Design review of the part built by this model. Coordinates are the model's own, in mm. Round coordinates to 2 decimals unless told otherwise and drop trailing zeros. One line per question, with ' | ' between items. Start each with the question number.
Item 1: Draft analysis for pull direction Z (two halves, no side actions). For faces 1 (the face through (-3, 7, 0)), 2 (the face through (-3, 7, -4.496)), state which applies: released by +Z, released by -Z, zero draft, split by the parting line, or undercut.
Item 2: Add section A-A, the plane z = -2.5. Give the number of separate pieces and of enclosed holes in the cut face, and give its area (3 significant figures).
Item 3: For L1, parallel to X at y = 142.5, z = -1.7; L2, parallel to Y at x = -160, z = -1.8; L3, parallel to X at y = 141.5, z = -2.8, list the stretches that pass through material, from the lowest coordinate up.
Autodesk Inventor part; units mm, degrees
ref_plane "YZ Plane" through (0, 0, 0) normal (1, 0, 0) x (0, 1, 0)
ref_plane "XZ Plane" through (0, 0, 0) normal (0, 1, 0) x (-1, 0, 0)
ref_plane "XY Plane" through (0, 0, 0) normal (0, 0, 1) x (1, 0, 0)
sketch "Sketch1" plane through (0, 0, 0) normal (0, 0, 1) x (1, 0, 0)
  line L0 (0, 316.484) -> (0, -316.484)
  line L1 (-334.6907, 0) -> (334.6907, 0)
  line L2 (239.0648, -226.06) -> (-239.0648, -226.06)
  line L3 (-239.0648, -226.06) -> (-239.0648, 226.06)
  line L4 (-239.0648, 226.06) -> (239.0648, 226.06)
  line L5 (239.0648, 226.06) -> (239.0648, -226.06)
  line L6 (239.0648, -226.06) -> (-239.0648, 226.06) construction
  line L7 (-239.0648, -226.06) -> (239.0648, 226.06) construction
  line L8 (220.345, -207.3402) -> (-220.345, -207.3402) construction
  line L9 (-220.345, -207.3402) -> (-220.345, 207.3402) construction
  line L10 (-220.345, 207.3402) -> (220.345, 207.3402) construction
  line L11 (220.345, 207.3402) -> (220.345, -207.3402) construction
  line L12 (220.345, -207.3402) -> (-220.345, 207.3402) construction
  line L13 (-220.345, -207.3402) -> (220.345, 207.3402) construction
  line L14 (-239.0648, -218.44) -> (239.0648, -218.44)
  line L15 (50.8, -191.06) -> (-50.8, -191.06)
  line L16 (-50.8, -191.06) -> (-50.8, -218.44)
  line L17 (-50.8, -218.44) -> (50.8, -218.44)
  line L18 (50.8, -218.44) -> (50.8, -191.06)
  line L19 (50.8, -191.06) -> (-50.8, -218.44) construction
  line L20 (-50.8, -191.06) -> (50.8, -218.44) construction
  point P0 (0, 0)
  point P1 (-156.5148, 207.3402)
  point P2 (0, 207.3402)
  point P3 (156.5148, 207.3402)
  point P4 (-156.5148, -207.3402)
  point P5 (0, -207.3402)
  point P6 (156.5148, -207.3402)
  point P7 (-220.345, 143.51)
  point P8 (-220.345, -143.51)
  point P9 (220.345, 143.51)
  point P10 (220.345, -117.0967)
  point P11 (-220.345, 0)
  point P12 (0, -218.44)
  point P13 (0, -226.06)
  point P14 (0, -204.75)
  point P15 (50.8, -218.44)
  dimension "d0" = 478.1296
  dimension "d1" = 452.12
  dimension "d3" = 18.7198
  dimension "d4" = 18.7198
  dimension "d7" = 143.51
  dimension "d8" = 143.51
  dimension "d10" = 82.55
  dimension "d20" = 82.55
  dimension "d21" = 82.55
  dimension "d23" = 7.62
  dimension "d24" = 35
  dimension "d25" = 101.6
extrude "Extrusion1" add sketch "Sketch1" against normal blind 4.4958 contours L4 L5 L1 L0 | L0 L1 L3 L4 | L1 L5 L14 L18 L15 L0 | L0 L15 L16 L14 L3 L1
hole "Hole1" at (-156.5148, 207.3402, 0) at (156.5148, 207.3402, 0) at (-156.5148, -207.3402, 0) at (156.5148, -207.3402, 0) at (220.345, 143.51, 0) at (220.345, -117.0967, 0) at (-220.345, 143.51, 0) at (-220.345, -143.51, 0) direction (0, 0, -1) diameter 8.255 end through all
fillet "Fillet1" radius 9.525 2 edges at (-239.0648, 226.06, -2.2479) (239.0648, 226.06, -2.2479)
fillet "Fillet2" radius 9.525 2 edges at (-239.0648, -218.44, -2.2479) (239.0648, -218.44, -2.2479)
fillet "Fillet3" radius 3.175 4 edges at (50.8, -191.06, -2.2479) (50.8, -218.44, -2.2479) (-50.8, -191.06, -2.2479) (-50.8, -218.44, -2.2479)
properties material "ACRYLIC, CLEAR"
Computed values:
1) face 1: released by +Z | face 2: released by -Z
2) separate pieces: 1 | enclosed holes: 8 | area: 209,000 mm^2
3) L1: x = -239.06 to -224.35, -216.34 to 216.34, 224.35 to 239.06 | L2: y = -218.44 to -209.55, -205.13 to 205.13, 209.55 to 226.06 | L3: x = -239.06 to -223.95, -216.74 to 216.74, 223.95 to 239.06
